Could you check a few things on this model? Use its own coordinates, in mm. Face numbers are marked on the shaded views. Coordinates: 2 decimals unless noted, no trailing zeros.
1) Will these pins go through, and if not, where does the flat tip stop? P1, Ø3, axis at y = -10, z = -10.5, coming from the -X side; P2, Ø1, axis at x = 18.5, z = -12, coming from the -Y side; P3, Ø4, axis at x = 38, z = -9.5, coming from the -Y side.
2) Thinking about a two-plate mould opening in X: for the marked faces 1, 2 and 3, which applies, released by +X, released by -X, zero draft, split by the parting line, or undercut?
3) If I drill on line 1 along Y through (x, z) = (0, -14.95); line 2 along Y through (x, z) = (0, -9.5); line 3 along Z through (x, y) = (-39, -37), over which ranges is the centre line in solid material (lowest first)?
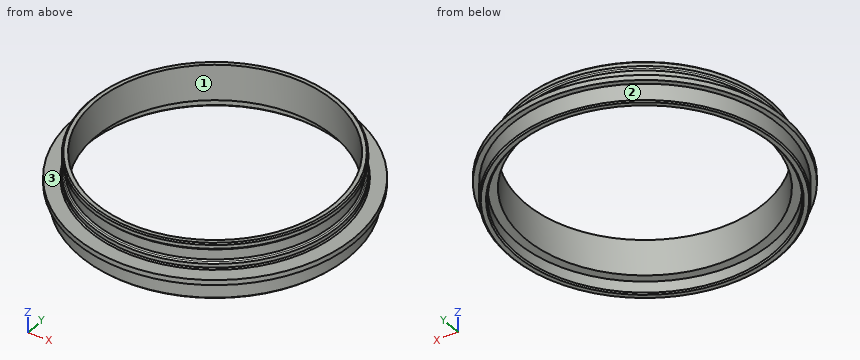
```python
from build123d import *

# Parameters (mm, degrees)
CHAMFER1_SIZE = 0.5


with BuildPart() as part:
    # Sketch1 → Revolve1 (revolve)
    with BuildSketch(Plane(origin=(0, 0, 0), x_dir=(1, 0, 0), z_dir=(0, 1, 0)), mode=Mode.PRIVATE) as revolve1_sk:
        Polygon((50.3, 19), (50.3, 14.1), (47, 14.1), (47, 0), (49, 0), (49, 2.5), (48, 2.5), (48, 7.5), (49, 7.5), (49, 10), (55, 10), (55, 12), (53, 12), (53, 19), align=None)
    revolve(revolve1_sk.sketch.rotate(Axis((0, 0, -69.169847328), (0, 0, 1)), 180), axis=Axis((0, 0, -69.169847328), (0, 0, 1)))

    # Chamfer1
    chamfer1_edges = [part.edges().sort_by_distance(p)[0] for p in [
        (49, 0, -10),
        (49, 0, -7.5),
        (48, 0, -7.5),
        (48, 0, -2.5),
        (49, 0, -2.5),
        (49, 0, 0),
        (50.3, 0, -19),
        (53, 0, -19),
    ]]
    chamfer(chamfer1_edges, length=CHAMFER1_SIZE - 0.0001)  # a hair under: the kernel refuses the full size


solid = part.part
```
Filled in:
1. P1: stops at x = -54.34
1. P2: stops at y = -51.97
1. P3: stops at y = -41.53
2. face 1: undercut
2. face 2: split by the parting line
2. face 3: zero draft
3. line 1: y = -53 to -50.3, 50.3 to 53
3. line 2: y = -49 to -47, 47 to 49
3. line 3: z = -12 to -10
